Input: dimensioned drawing with shaded views. Units: mm. Origin: part minimum x, y, z. Coordinates: 2 decimals unless noted, no trailing zeros. Order: outer loops, then holes, each group sorted by start corner. A loop starts at its lowest first (then second) coordinate and runs counter-clockwise, first axis right, second up. Notation, with made-up numbers: (40, 0) -> (61, 0) arc R21 cw to (61, 36) -> close; hole circle Ø7 at (-20.75, -7). An arc over 180 degrees is marked (long way). Answer in a Markdown table with one row per item. Add a question column.
1) Ray query, line 1 (X direction, y = 5.75, z = 76.2); line 2 (Z direction, x = 76.2, y = 3). Return the intervals inside material, ascending. Write a range as from..to.
2) Section query B-B on x = 196.85. Return the cut outline in (y, z), then the cut area to 3 significant figures.
3) Contact query for a flat-ended pin moving along its axis: P1, Ø1, axis at x = 189.5, z = 65, coming from the -Y side. Output: stop coordinate, or through.
4) Section query C-C on x = 76.2. Return the cut outline in (y, z), then the cut area to 3 significant figures.
5) Section query A-A on z = 76.2. Return the cut outline in (x, y).
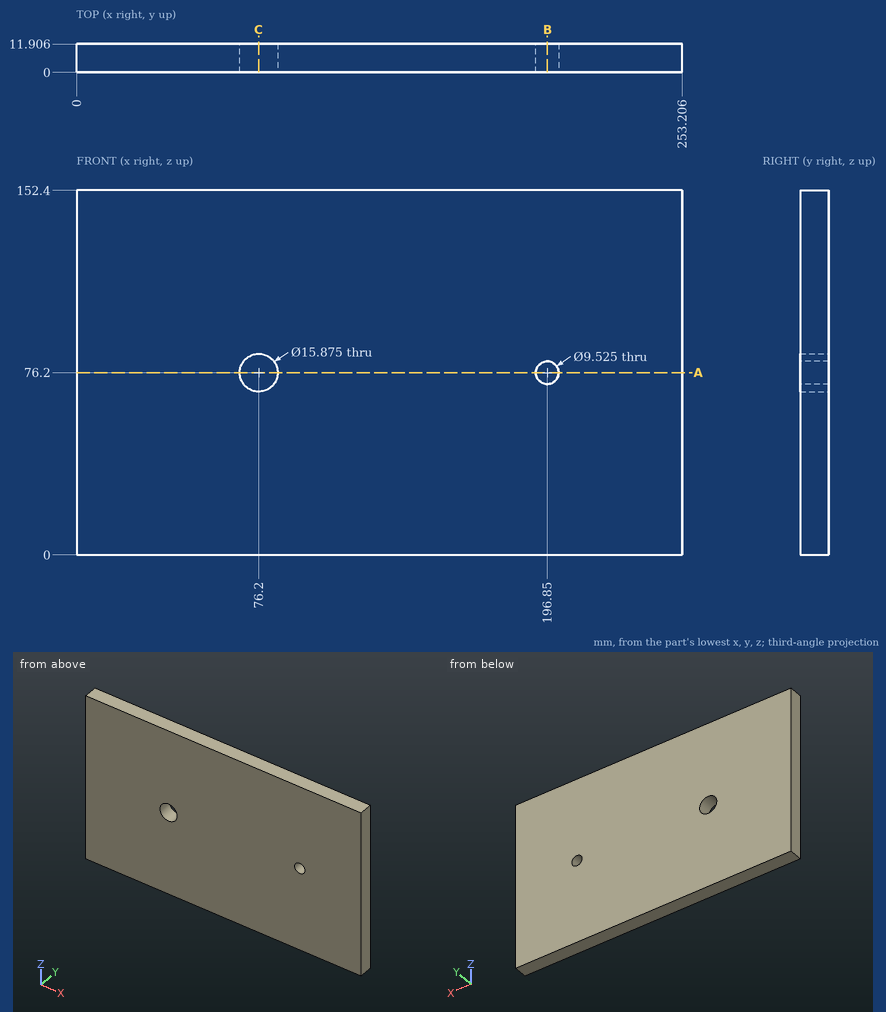
Result:
| question | item | result |
|---|---|---|
| 1 | line 1 | 0..68.26, 84.14..192.09, 201.61..253.21 |
| 1 | line 2 | 0..68.26, 84.14..152.4 |
| 2 | outline | (0, 0) -> (11.91, 0) -> (11.91, 71.44) -> (0, 71.44) -> close; (0, 80.96) -> (11.91, 80.96) -> (11.91, 152.4) -> (0, 152.4) -> close |
| 2 | area | 1,700 mm2 |
| 3 | P1 | y = 0 |
| 4 | outline | (0, 0) -> (11.91, 0) -> (11.91, 68.26) -> (0, 68.26) -> close; (0, 84.14) -> (11.91, 84.14) -> (11.91, 152.4) -> (0, 152.4) -> close |
| 4 | area | 1,630 mm2 |
| 5 | outline | (0, 0) -> (68.26, 0) -> (68.26, 11.91) -> (0, 11.91) -> close; (84.14, 0) -> (192.09, 0) -> (192.09, 11.91) -> (84.14, 11.91) -> close; (201.61, 0) -> (253.21, 0) -> (253.21, 11.91) -> (201.61, 11.91) -> close |
